Check sheet for the modelled part. Datum: model origin and axes. Units: mm. A direction names the side the tool comes from. Coordinates: 2 decimals unless noted, no trailing zeros. Loops run counter-clockwise (first coordinate to the right, second up) from the corner with the lowest first, then second, coordinate; pieces in that order, holes last. Notation, with made-up numbers: M -3.5,32.5 L 55.5,32.5 A18 ccw 55.5,54.5 Z; hole C 39,59.5 d11. An arc over 180 degrees is marked long. Return JSON: item names as keys, results as strings.
from build123d import *

# Parameters (mm, degrees)
F0_W     = 160
F0_H     = 95
F1_DEPTH = 8
F2_W     = 153.534181416
F2_H     = 89.7976644337
F3_DEPTH = 3
F4_W     = 75.6339989603
F4_H     = 27.7607943863
F5_DEPTH = 16
F6_R     = 5


with BuildPart() as f1:
    # F0 (on Front) → F1 (new body)
    with BuildSketch(Plane.XZ):
        with Locations((4.0975642204, 18.1421419978)):
            Rectangle(F0_W, F0_H)
    extrude(amount=F1_DEPTH)

    # F2 (on face) → F3 (cut)
    with BuildSketch(Plane.XZ.offset(8)):
        with Locations((3.6726556718, 18.1294959038)):
            Rectangle(F2_W, F2_H)
    extrude(amount=-F3_DEPTH, mode=Mode.SUBTRACT)

    # F4 (on face) → F5 (join)
    with BuildSketch(Plane(origin=(0, 0, 0), x_dir=(-1, 0, 0), z_dir=(0, 1, 0))):
        with Locations((-5.2306558937, 21.3871421292)):
            Rectangle(F4_W, F4_H)
    extrude(amount=F5_DEPTH)

    # F6
    f6_edges = [f1.edges().sort_by_distance(p)[0] for p in [
        (-32.586344, 8, 35.267539),
        (43.047655, 8, 35.267539),
        (5.230656, 0, 35.267539),
        (5.230656, 16, 35.267539),
        (43.047655, 8, 7.506745),
        (-32.586344, 8, 7.506745),
        (5.230656, 0, 7.506745),
        (5.230656, 16, 7.506745),
        (-32.586344, 0, 21.387142),
        (43.047655, 0, 21.387142),
    ]]
    fillet(f6_edges, radius=F6_R)


solid = f1.part
1) Section check C-C on y = 7.75. Record the cut outline in (x, z).
Answers:
{"outline": "M -32.59,12.51 A5 ccw -27.59,7.51 L 38.05,7.51 A5 ccw 43.05,12.51 L 43.05,30.27 A5 ccw 38.05,35.27 L -27.59,35.27 A5 ccw -32.59,30.27 Z"}
2) Section check D-D on x = 28. Record the cut outline in (y, z), then the cut area to 3 significant figures.
Answers:
{"outline": "M -8,-29.36 L 0,-29.36 L 0,2.51 A5 cw 5,7.51 L 11,7.51 A5 ccw 16,12.51 L 16,30.27 A5 ccw 11,35.27 L 5,35.27 A5 cw 0,40.27 L 0,65.64 L -8,65.64 L -8,63.03 L -5,63.03 L -5,-26.77 L -8,-26.77 Z", "area": "935 mm²"}
3) Scan lines: line 1 along Z through (x, y) = (-55, -6); line 2 along Y through (x, z) = (-21, -21.5); line 3 along X through (y, z) = (-6.5, -8.5). Record each from-to range of solid material in increasing order. Write a range as [from, to].
Answers:
{"line 1": "[-29.36, -26.77], [63.03, 65.64]", "line 2": "[-5, 0]", "line 3": "[-75.9, -73.09], [80.44, 84.1]"}
4) Draft check along X on faces 1 (the face through (3, -7, -26.769)), 2 (the face through (43.048, 10, 21)), 3 (the face through (4.7, 14.5, 33.84)). Enter one of: +X half, -X half, draft (parallel to the pull), parting line (faces both ways), or undercut.
Answers:
{"face 1": "undercut", "face 2": "+X half", "face 3": "draft"}
5) Go/stop test with flat-tipped pins: pin 1 Ø5 at (x, y) = (-2.5, 7) entering from -Z; pin 2 Ø3 at (x, y) = (21, 7.5) entering from +Z; pin 3 Ø12 at (x, z) = (-28.5, 41.5) entering from -Y. Record where each tip stops, or that it passes through.
Answers:
{"pin 1": "z = 7.48", "pin 2": "z = 35.27", "pin 3": "y = -5"}
6) Section check A-A on z = 15.5. Record the cut outline in (x, y).
Answers:
{"outline": "M -75.9,-8 L -73.09,-8 L -73.09,-5 L 80.44,-5 L 80.44,-8 L 84.1,-8 L 84.1,0 L 48.05,0 A5 cw 43.05,5 L 43.05,16 L -32.59,16 L -32.59,5 A5 cw -37.59,0 L -75.9,0 Z"}
7) Section check B-B on x = 64.5. Record the cut outline in (y, z).
Answers:
{"outline": "M -8,-29.36 L 0,-29.36 L 0,65.64 L -8,65.64 L -8,63.03 L -5,63.03 L -5,-26.77 L -8,-26.77 Z"}
8) Set-up check for faces 4 (the face through (41.62, 9.35, 9.01)), 5 (the face through (-32.586, 10, 21)), 6 (the face through (3, -7, 63.028)), 7 (the face through (-31.083, 9.355, 33.842)): record each of +Z, -Z, +X, -X, +Y, -Y from which the full face is reachable in a straight line by a thin tool's end or side.
Answers:
{"face 4": "-Z, +X, +Y", "face 5": "+Z, -Z, -X, +Y", "face 6": "-Y", "face 7": "+Z, -X, +Y"}
